```python
from build123d import *

# Parameters (mm, degrees)
SKETCH_1_R      = 3
SKETCH_1_R_2    = 2.5
EXTRUDE_1_DEPTH = 71.5
SKETCH_2_R      = 3
SKETCH_2_R_2    = 1
EXTRUDE_2_DEPTH = 1
SKETCH_3_R      = 2.5
EXTRUDE_3_DEPTH = 1.5
SKETCH_4_R      = 1.4
SKETCH_4_R_2    = 1
EXTRUDE_4_DEPTH = 9
SKETCH_5_R      = 1.4
SKETCH_5_R_2    = 0.25
EXTRUDE_5_DEPTH = 1
SKETCH_6_R      = 0.35
SKETCH_6_R_2    = 0.25
EXTRUDE_6_DEPTH = 20


with BuildPart() as part:
    # 草图1 → 凸台-拉伸1 (new body)
    with BuildSketch(Plane.XY):
        Circle(SKETCH_1_R)
        Circle(SKETCH_1_R_2, mode=Mode.SUBTRACT)
    extrude(amount=EXTRUDE_1_DEPTH)

    # 草图2 → 凸台-拉伸2 (add)
    with BuildSketch(Plane.XY.offset(71.5)):
        Circle(SKETCH_2_R)
        with Locations((1.174015937, 0)):
            Circle(SKETCH_2_R_2, mode=Mode.SUBTRACT)
    extrude(amount=-EXTRUDE_2_DEPTH)

    # 草图3 → 凸台-拉伸3 (add)
    with BuildSketch(Plane(origin=(0, 0, 0), x_dir=(-1, 0, 0), z_dir=(0, 0, -1))):
        with BuildLine():
            Line((7.298274993, -1.719289065), (0.894824979, -3.720367194))
            ThreePointArc((0.894824979, -3.720367194), (0, -3.85692726), (-0.894824979, -3.720367194))
            Line((-0.894824979, -3.720367194), (-7.298274993, -1.719289065))
            ThreePointArc((-7.298274993, -1.719289065), (-7.805690695, -1.357145565), (-8, -0.764809087))
            Line((-8, -0.764809087), (-8, 0))
            Line((-8, 0), (-8, 0.764809087))
            ThreePointArc((-8, 0.764809087), (-7.805690695, 1.357145565), (-7.298274993, 1.719289065))
            Line((-7.298274993, 1.719289065), (-0.894824979, 3.720367194))
            ThreePointArc((-0.894824979, 3.720367194), (0, 3.85692726), (0.894824979, 3.720367194))
            Line((0.894824979, 3.720367194), (7.298274993, 1.719289065))
            ThreePointArc((7.298274993, 1.719289065), (7.805690695, 1.357145565), (8, 0.764809087))
            Line((8, 0.764809087), (8, 0))
            Line((8, 0), (8, -0.764809087))
            ThreePointArc((8, -0.764809087), (7.805690695, -1.357145565), (7.298274993, -1.719289065))
        make_face()
        Circle(SKETCH_3_R, mode=Mode.SUBTRACT)
    extrude(amount=EXTRUDE_3_DEPTH)

    # 草图4 → 凸台-拉伸4 (add)
    with BuildSketch(Plane.XY.offset(71.5)):
        with Locations((1.174015937, 0)):
            Circle(SKETCH_4_R)
        with Locations((1.174015937, 0)):
            Circle(SKETCH_4_R_2, mode=Mode.SUBTRACT)
    extrude(amount=EXTRUDE_4_DEPTH)

    # 草图5 → 凸台-拉伸5 (add)
    with BuildSketch(Plane.XY.offset(80.5)):
        with Locations((1.174015937, 0)):
            Circle(SKETCH_5_R)
        with Locations((1.74042038, 0)):
            Circle(SKETCH_5_R_2, mode=Mode.SUBTRACT)
    extrude(amount=EXTRUDE_5_DEPTH)

    # 草图6 → 凸台-拉伸6 (add)
    with BuildSketch(Plane.XY.offset(81.5)):
        with Locations((1.74042038, 0)):
            Circle(SKETCH_6_R)
        with Locations((1.74042038, 0)):
            Circle(SKETCH_6_R_2, mode=Mode.SUBTRACT)
    extrude(amount=EXTRUDE_6_DEPTH)


solid = part.part
```
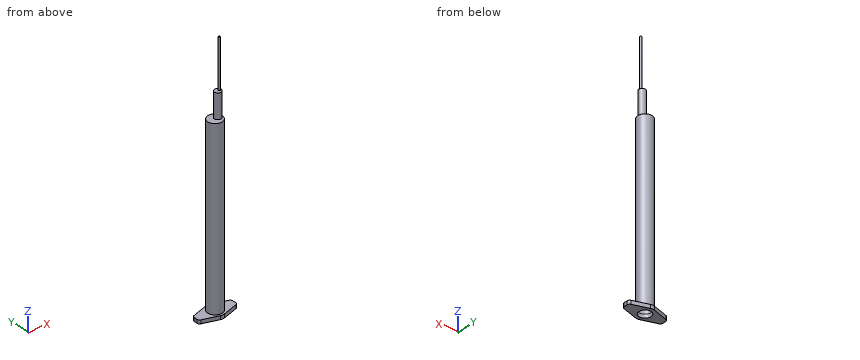
Model file for the job. Use its own axes, mm. Round coordinates to 2 decimals unless told otherwise and drop trailing zeros. Loops run counter-clockwise (first coordinate to the right, second up) from the corner with the lowest first, then second, coordinate; pieces in that order, holes last. Notation, with made-up numbers: M 18,42.25 L 33,42.25 A17 ccw 33,61.25 Z; hole C -5,14 d6. An arc over 180 degrees is marked long. Put each result on its own line as item: value. Start each with the question number.
Item 1: Cut at B-B (z = 88.5). List the corners of the cut face in (x, y).
Item 2: Drill centre lines: line 1 along X through (y, z) = (0, -0.8); line 2 along X through (y, z) = (-0.25, 61); line 3 along Y through (x, z) = (0, 55). Where is each one in solid material? Low to high.
Item 3: Drop flat-ended pins along their axis: P1, Ø0.6, axis at x = 1, y = 0.5, coming from the -Z side; P2, Ø1.5, axis at x = -3.5, z = 41.5, coming from the -Y side; P3, Ø3, axis at x = 0, y = 0, coming from the -Z side. Give the stop position or say it passes through.
Item 4: Cut at A-A (z = 15.5). List the corners of the cut face in (x, y).
Answer block:
1. outline: C 1.74,0 d0.7; hole C 1.74,0 d0.5
2. line 1: -8 to -2.5, 2.5 to 8
2. line 2: -2.99 to -2.49, 2.49 to 2.99
2. line 3: -3 to -2.5, 2.5 to 3
3. P1: z = 80.5
3. P2: y = -1.2
3. P3: z = 70.5
4. outline: C 0,0 d6; hole C 0,0 d5
